Check sheet for the drawn part. Datum: minimum x, y, z corner. Units: mm. A direction names the side the tool comes from. Give positions to 0.01 mm unless a question says otherwise; leave off trailing zeros. Loops run counter-clockwise (first coordinate to the right, second up) from the corner with the lowest first, then second, coordinate; pieces in that order, holes last. Notation, with made-up numbers: (28, 87.5) - (40, 87.5) arc R30 ccw to (40, 118.5) - close; hole circle Ø8 at (-17, -11.5). An arc over 180 degrees is marked (long way). Use a Markdown table: item, result. Add a question column.
1. Set-up check for the marked faces 1 and 2: record each of +Z, -Z, +X, -X, +Y, -Y from which the full face is reachable in a straight line by a thin tool's end or side.
2. Cross-section at B-B on x = 35.5. Enter the section's corners in (y, z).
3. Material ranges on L1, parallel to X at y = 45.5, z = 33.5; L2, parallel to Y at x = 25, z = 34; L3, parallel to Z at x = 148.5, y = 6, recorded low to high.
4. Cross-section at C-C on y = 60.5. Enter the section's corners in (x, z).
5. Draft check along Y on the marked faces 3, 4 and 5. Enter one of: pulls with the +Y half, pulls with the -Y half, needs draft (parallel to the pull), parting line crosses it, or undercut.
6. Depth check by flat-ended pin: P1, Ø5, axis at x = 111, y = 64, coming from the +Z side. Enter the tip coordinate at first touch or a pass-through.
7. Cross-section at A-A on z = 30. Enter the section's corners in (x, y).
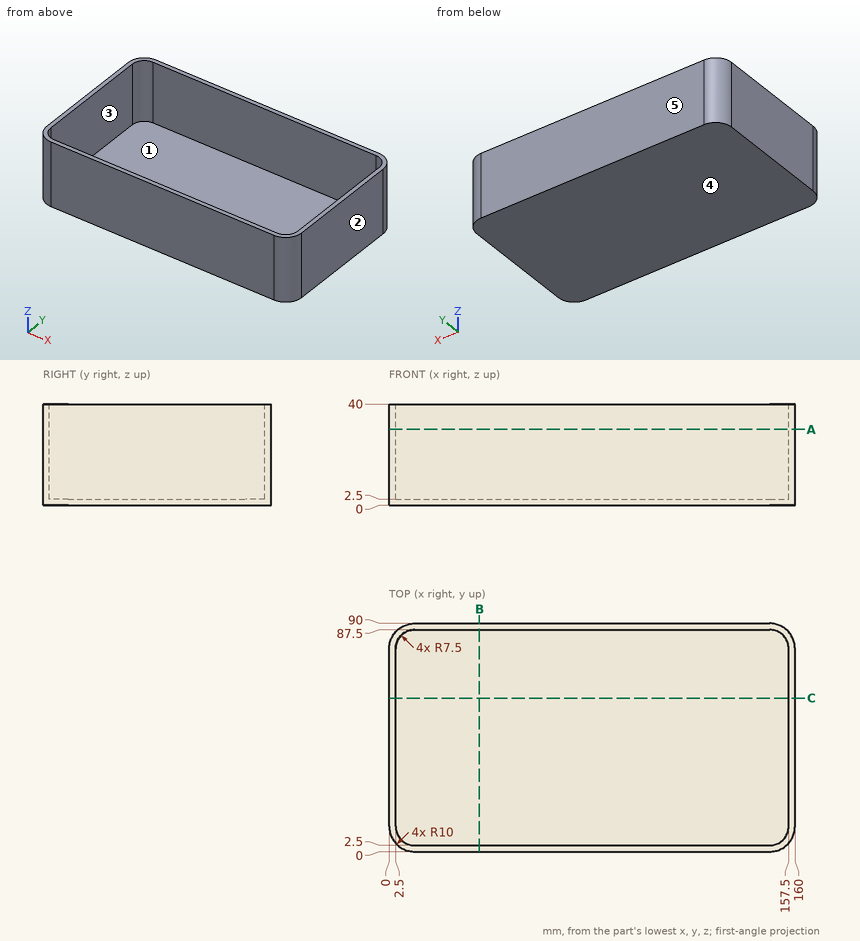
Values found:
| question | item | result |
|---|---|---|
| 1 | face 1 | +Z |
| 1 | face 2 | +Z, -Z, +X, +Y, -Y |
| 2 | outline | (0, 0) - (90, 0) - (90, 40) - (87.5, 40) - (87.5, 2.5) - (2.5, 2.5) - (2.5, 40) - (0, 40) - close |
| 3 | L1 | x = 0 to 2.5, 157.5 to 160 |
| 3 | L2 | y = 0 to 2.5, 87.5 to 90 |
| 3 | L3 | z = 0 to 2.5 |
| 4 | outline | (0, 0) - (160, 0) - (160, 40) - (157.5, 40) - (157.5, 2.5) - (2.5, 2.5) - (2.5, 40) - (0, 40) - close |
| 5 | face 3 | undercut |
| 5 | face 4 | needs draft |
| 5 | face 5 | pulls with the +Y half |
| 6 | P1 | stops at z = 2.5 |
| 7 | outline | (0, 10) arc R10 ccw to (10, 0) - (150, 0) arc R10 ccw to (160, 10) - (160, 80) arc R10 ccw to (150, 90) - (10, 90) arc R10 ccw to (0, 80) - close; hole (2.5, 10) arc R7.5 ccw to (10, 2.5) - (150, 2.5) arc R7.5 ccw to (157.5, 10) - (157.5, 80) arc R7.5 ccw to (150, 87.5) - (10, 87.5) arc R7.5 ccw to (2.5, 80) - close |
